```python
from build123d import *

# Parameters (mm, degrees)
SALIENTE_EXTRUIR1_DEPTH   = 7.5
SALIENTE_EXTRUIR1_2_DEPTH = 7.5
SALIENTE_EXTRUIR2_DEPTH   = 14
CROQUIS4_W                = 52.808095268
CROQUIS4_H                = 22
CROQUIS4_W_2              = 47.625032345
CROQUIS4_H_2              = 2.85152228
SALIENTE_EXTRUIR3_DEPTH   = 1.2


with BuildPart() as part:
    # Croquis2 → Saliente-Extruir1 (new body)
    with BuildSketch(Plane(origin=(0, -12.4, 0), x_dir=(1, 0, 0), z_dir=(0, 1, 0))):
        with BuildLine():
            Line((20.9, 0), (20.9, 8.468551509))
            ThreePointArc((20.9, 8.468551509), (14.039862076, 2.13695997), (5.744958612, 6.420080362))
            Line((5.744958612, 6.420080362), (5.788277469, 0))
            Line((5.788277469, 0), (20.9, 0))
        make_face()
    extrude(amount=SALIENTE_EXTRUIR1_DEPTH)



with BuildPart() as body_2:
    # Croquis2 → Saliente-Extruir1 2 (new body)
    with BuildSketch(Plane(origin=(0, -12.4, 0), x_dir=(1, 0, 0), z_dir=(0, 1, 0))):
        with BuildLine():
            ThreePointArc((-20.9, 8.468551509), (-14.039862076, 2.13695997), (-5.744958612, 6.420080362))
            Line((-5.744958612, 6.420080362), (-5.788277469, 0))
            Line((-5.788277469, 0), (-20.9, 0))
            Line((-20.9, 0), (-20.9, 8.468551509))
        make_face()
    extrude(amount=SALIENTE_EXTRUIR1_2_DEPTH)


with BuildPart() as body_3:
    # Croquis3 → Saliente-Extruir2 (new body)
    with BuildSketch(Plane.XY):
        Polygon((24.404047634, 4.6), (24.404047634, 1.902402318), (24.404047634, -1.452453504), (22.804047634, -1.452453504), (22.804047634, 1.902402318), (-22.804047634, 1.902402318), (-22.804047634, -1.452453504), (-24.404047634, -1.452453504), (-24.404047634, 1.902402318), (-24.404047634, 4.6), (-6.312940469, 4.6), (-6.312940469, 6.117496706), (5.744958612, 6.117496706), (5.744958612, 4.6), align=None)
    extrude(amount=-SALIENTE_EXTRUIR2_DEPTH)


with BuildPart() as part_1:
    add(part.part)

    add(body_2.part)  # Saliente-Extruir3 merges body 2

    add(body_3.part)  # Saliente-Extruir3 merges body 3
    # Croquis4 → Saliente-Extruir3 (add)
    with BuildSketch(Plane.XY):
        with Locations((0, -3.4)):
            Rectangle(CROQUIS4_W, CROQUIS4_H)
        with Locations((0.009244494, -3.943262508)):
            Rectangle(CROQUIS4_W_2, CROQUIS4_H_2, mode=Mode.SUBTRACT)
    extrude(amount=SALIENTE_EXTRUIR3_DEPTH)


solid = part_1.part
```
Geometry: final body of the model. Coordinates: model frame, mm. A direction names the side the tool comes from. Coordinates: 2 decimals unless noted, no trailing zeros. Order: outer loops, then holes, each group sorted by start corner. A loop starts at its lowest first (then second) coordinate and runs counter-clockwise, first axis right, second up. Notation, with made-up numbers: M 59,75.5 L 85,75.5 A28 ccw 85,108.5 Z; hole C -30.5,75 d1. An arc over 180 degrees is marked long. Answer as CSV lines item,"result".
Q1. Section D-D on y = 3. Return the cut outline in (x, z), and give its area (3 significant figures).
Answers:
outline,"M -26.4,0 L -24.4,0 L -24.4,-14 L 24.4,-14 L 24.4,0 L 26.4,0 L 26.4,1.2 L -26.4,1.2 Z"
area,"747 mm^2"
Q2. Section B-B on x = -5. Return the cut outline in (y, z), and give its area (3 significant figures).
Answers:
outline,"M -14.4,0 L -5.37,0 L -5.37,1.2 L -14.4,1.2 Z; M -2.52,0 L 1.9,0 L 1.9,-14 L 6.12,-14 L 6.12,0 L 7.6,0 L 7.6,1.2 L -2.52,1.2 Z"
area,"82.0 mm^2"
Q3. Section C-C on z = -12.25. Return the cut outline in (x, y).
Answers:
outline,"M -24.4,-1.45 L -22.8,-1.45 L -22.8,1.9 L 22.8,1.9 L 22.8,-1.45 L 24.4,-1.45 L 24.4,4.6 L 5.74,4.6 L 5.74,6.12 L -6.31,6.12 L -6.31,4.6 L -24.4,4.6 Z"
Q4. Section A-A on y = -3.5. Return the cut outline in (x, z), and give its area (3 significant figures).
Answers:
outline,"M -26.4,0 L -23.8,0 L -23.8,1.2 L -26.4,1.2 Z; M 23.82,0 L 26.4,0 L 26.4,1.2 L 23.82,1.2 Z"
area,"6.22 mm^2"
Q5. Draft query along X for faces 1 (the flat face through (-22.804, 0, -7)), 2 (the flat face through (24.404, 2, -7)), 3 (the flat face through (0, -2.518, 1)), 4 (the flat face through (13, -4.9, -1)). Return one class per face: pulls with the +X half, pulls with the -X half, needs draft (parallel to the pull), parting line crosses it, or undercut.
Answers:
face 1,"undercut"
face 2,"pulls with the +X half"
face 3,"undercut"
face 4,"needs draft"
Q6. First-contact query: P1, Ø1.7, axis at y = 5.5, z = -5.5, coming from the +X side; P2, Ø3, axis at x = -0.5, y = -7, coming from the -Z side; P3, Ø4, axis at x = -16, z = -4, coming from the -Y side. Flat tips, straight axial feed; report the tip coordinate or a pass-through.
Answers:
P1,"stops at x = 5.74"
P2,"stops at z = 0"
P3,"stops at y = -12.4"
Q7. Set-up query: faces 5 (the flat face through (22.804, 0, -7)), 6 (the flat face through (-24.404, 2, -7)), 7 (the flat face through (-13, -12.4, -1)). Return all of +Z, -Z, +X, -X, +Y, -Y with unobstructed straight access to the full face (end or side cutting, diameter ignored); none if empty.
Answers:
face 5,"-Z, -Y"
face 6,"-Z, -X, +Y, -Y"
face 7,"-Z, +X, -X, -Y"
Q8. Line query: probe 1 along Y at (x, z) = (-10, -1.5); probe 2 along X at (y, z) = (-8.75, -1.75); probe 3 along Y at (x, z) = (23, 0.5). Output: solid intervals per line, ascending. Write a range as [from, to].
Answers:
probe 1,"y = [-12.4, -4.9], [1.9, 4.6]"
probe 2,"x = [-20.9, -5.78], [5.78, 20.9]"
probe 3,"y = [-14.4, -5.37], [-2.52, 7.6]"
